Study the drawing (mm; zero at the part's minimum x, y, z) and answer. Coordinates: 2 decimals unless noted, no trailing zeros. Loops run counter-clockwise (first coordinate to the right, second up) from the corner with the lowest first, then second, coordinate; pieces in that order, holes last. Notation, with made-up numbers: (73, 9) -> (96, 9) arc R17 cw to (96, 21) -> close; hole circle Ø7 at (43, -35). An arc over 180 degrees is marked (long way). One line per question, with ' | ' between items. Start each with the question number.
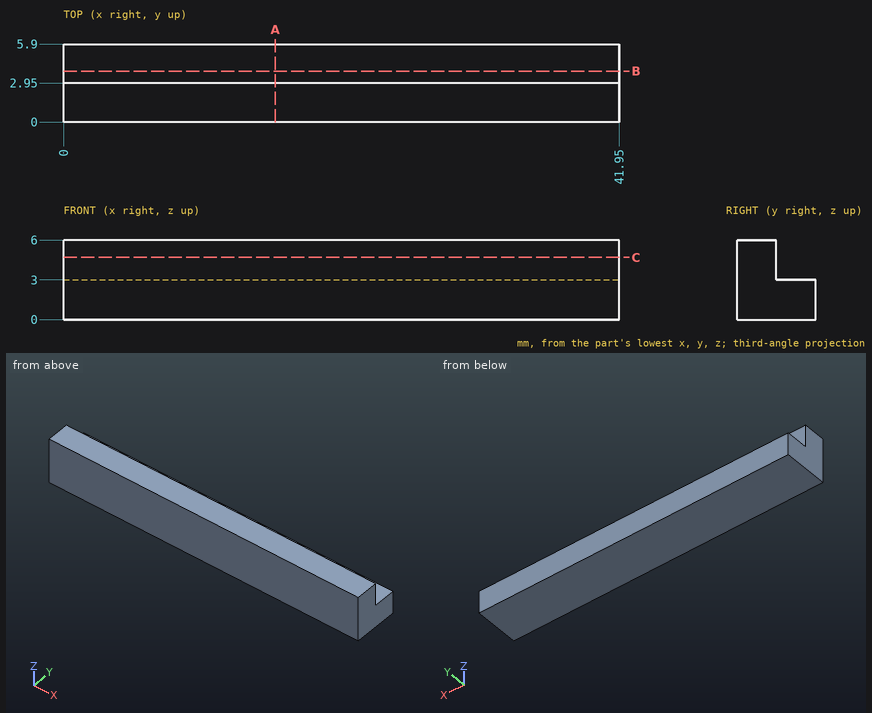
(1) Each of these flat-tipped pins is pushed along its axis until it touches: pin 1 Ø3.5 at (x, z) = (16, 5) entering from +Y; pin 2 Ø3 at (x, y) = (12, 4) entering from +Z. Where does it stop, or does it pass through?
(2) Section A-A on x = 16 is taken. Write down the section's boundary in (y, z), plus the area to 4 significant figures.
(3) Find the intervals of material crossed by probe 1 along Y at (x, z) = (26, 4.7); probe 2 along Z at (x, y) = (13, 5.05), in increasing order. Write a range as from..to.
(4) Section C-C on z = 4.7 is taken. Write down the section's boundary in (x, y).
(5) Section B-B on y = 3.85 is taken. Write down the section's boundary in (x, z), plus the area to 3 significant figures.
Working result:
1) pin 1: stops at y = 2.95 | pin 2: stops at z = 6
2) outline: (0, 0) -> (5.9, 0) -> (5.9, 3) -> (2.95, 3) -> (2.95, 6) -> (0, 6) -> close | area: 26.55 mm2
3) probe 1: y = 0..2.95 | probe 2: z = 0..3
4) outline: (0, 0) -> (41.95, 0) -> (41.95, 2.95) -> (0, 2.95) -> close
5) outline: (0, 0) -> (41.95, 0) -> (41.95, 3) -> (0, 3) -> close | area: 126 mm2
